Here's how the part is built. I have some questions about the finished solid (model axes, mm). Face numbers are marked on the shaded views. A direction names the side the tool comes from. Coordinates: 2 decimals unless noted, no trailing zeros. Order: outer loops, then holes, each group sorted by start corner. A loop starts at its lowest first (then second) coordinate and runs counter-clockwise, first axis right, second up. Notation, with made-up numbers: (81.25, -35) - (110.25, -35) arc R21 cw to (110.25, -29) - close; hole circle Ø4 at (17.5, 69). An arc over 180 degrees is marked (long way). Answer as CSV lines item,"result". Start each with the question number.
Q1. For pin 1 Ø1.2 at (y, z) = (0.5, 4) entering from -X; pin 2 Ø2.5 at (y, z) = (-3.5, 6) entering from +X (3 decimals); pin 3 Ø3.5 at (y, z) = (-3, 1.5) entering from -X (3 decimals), each with a flat end and sliding along its axis, tell me the tip position at first contact or that it passes through.
Q2. Suppose I cut it at D-D (x = 1.5). Please give me the cut outline in (y, z), then the cut area to 3 significant figures.
Q3. Suppose I cut it at A-A (x = 18.5). Please give me the cut outline in (y, z) (3 decimals), then the cut area to 3 significant figures.
Q4. Suppose I cut it at B-B (z = 4). Please give me the cut outline in (x, y).
Q5. I need wall thicknesses on line 1 (Y direction, x = 18.5, z = 1.25); line 2 (X direction, y = 8, z = 5); line 3 (Z direction, x = 13.25, y = 3.5) (3 decimals). Which ranges of each line are inside material? Lowest first, please.
Q6. Suppose I cut it at C-C (y = 1). Please give me the cut outline in (x, z), then the cut area to 3 significant figures.
Q7. For the marked faces 1, 2 and 3, which set-ups out of +Z, -Z, +X, -X, +Y, -Y let a thin tool reach every point of the face, with its end or its side?
Q8. Thinking about a two-plate mould opening in Y: for the marked faces 4, 5 and 6, which applies, released by +Y, released by -Y, zero draft, split by the parting line, or undercut?
Autodesk Inventor part; units mm, degrees
ref_plane "YZ Plane" through (0, 0, 0) normal (1, 0, 0) x (0, 1, 0)
ref_plane "XZ Plane" through (0, 0, 0) normal (0, 1, 0) x (-1, 0, 0)
ref_plane "XY Plane" through (0, 0, 0) normal (0, 0, 1) x (1, 0, 0)
sketch "Sketch1" plane through (0, 0, 0) normal (0, 0, 1) x (1, 0, 0)
  line L0 (0, 0) -> (25, 0)
  line L1 (25, 0) -> (25, 12)
  line L2 (25, 12) -> (0, 12)
  line L3 (0, 12) -> (0, 0)
  line L4 (10.625, 0) -> (14.375, 0)
  line L5 (14.375, 0) -> (14.375, -6)
  line L6 (14.375, -6) -> (10.625, -6) construction
  line L7 (10.625, -6) -> (10.625, 0)
  line L8 (0, -6) -> (25, -6)
  line L9 (25, -6) -> (25, -9)
  line L10 (25, -9) -> (0, -9)
  line L11 (0, -9) -> (0, -6)
  point P0 (14.375, 0)
  dimension "d0" = 25
  dimension "d1" = 12
  dimension "d2" = 6
  dimension "d3" = 3.75
  dimension "d4" = 10.625
  dimension "d28" = 0
  dimension "d29" = 3
extrude "Extrusion1" add sketch "Sketch1" along normal blind 8
sketch "Sketch2" plane through (0, 12, 0) normal (0, 1, 0) x (1, 0, 0)
  line L0 (0, 0) -> (10.625, 0)
  line L1 (0, 0) -> (25, 0)
  line L2 (25, 0) -> (25, -8)
  line L3 (25, -8) -> (0, -8)
  line L4 (0, -8) -> (0, 0)
  line L5 (2.75, -1.875) -> (22.25, -1.875)
  line L6 (22.25, -1.875) -> (22.25, -6.125)
  line L7 (22.25, -6.125) -> (2.75, -6.125)
  line L8 (2.75, -6.125) -> (2.75, -1.875)
  line L9 (5.05, -4.75) -> (10.8, -4.75)
  line L10 (10.8, -4.75) -> (10.8, -3.25)
  line L11 (10.8, -3.25) -> (5.05, -3.25)
  line L12 (5.05, -3.25) -> (5.05, -4.75)
  line L13 (14.2, -4.75) -> (19.95, -4.75)
  line L14 (19.95, -4.75) -> (19.95, -3.25)
  line L15 (19.95, -3.25) -> (14.2, -3.25)
  line L16 (14.2, -3.25) -> (14.2, -4.75)
  line L17 (2.95, -6) -> (22.05, -6) construction
  line L18 (22.05, -6) -> (22.05, -2) construction
  line L19 (22.05, -2) -> (2.95, -2) construction
  line L20 (2.95, -2) -> (2.95, -6) construction
  dimension "d7" = 25
  dimension "d8" = 8
  dimension "d9" = 19.5
  dimension "d10" = 4.25
  dimension "d11" = 1.875
  dimension "d12" = 2.75
  dimension "d13" = 1.5
  dimension "d14" = 19.1
  dimension "d15" = 4
  dimension "d16" = 2.95
  dimension "d17" = 2
  dimension "d18" = 2.1
  dimension "d20" = 2.1
  dimension "d21" = 1.25
  dimension "d22" = 5.75
  dimension "d23" = 5.75
extrude "Extrusion2" cut sketch "Sketch2" against normal blind 10 contours L5 L6 L7 L8 | L12 L11 L10 L9 | L16 L15 L14 L13
extrude "Extrusion3" cut sketch "Sketch2" against normal blind 18 contours L12 L11 L10 L9 | L16 L15 L14 L13
properties part number "fusebox"
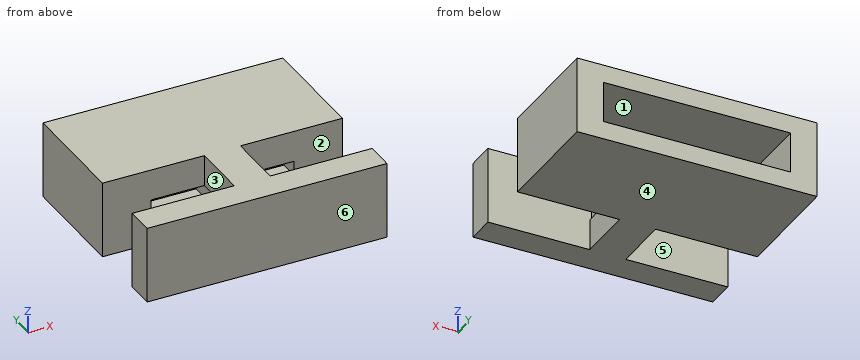
Here are the results:
1,pin 1,"stops at x = 0"
1,pin 2,"stops at x = 14.375"
1,pin 3,"stops at x = 10.625"
2,outline,"(-9, 0) - (-6, 0) - (-6, 8) - (-9, 8) - close; (0, 0) - (12, 0) - (12, 8) - (0, 8) - close"
2,area,"120 mm²"
3,outline,"(-9, 0) - (-6, 0) - (-6, 8) - (-9, 8) - close; (0, 0) - (12, 0) - (12, 1.875) - (2, 1.875) - (2, 3.25) - (0, 3.25) - close; (0, 4.75) - (2, 4.75) - (2, 6.125) - (12, 6.125) - (12, 8) - (0, 8) - close"
3,area,"74.5 mm²"
4,outline,"(0, -9) - (25, -9) - (25, -6) - (14.2, -6) - (14.2, 2) - (10.8, 2) - (10.8, -6) - (0, -6) - close; (0, 0) - (5.05, 0) - (5.05, 2) - (2.75, 2) - (2.75, 12) - (0, 12) - close; (19.95, 0) - (25, 0) - (25, 12) - (22.25, 12) - (22.25, 2) - (19.95, 2) - close"
5,line 1,"y = -9 to -6, 0 to 12"
5,line 2,"x = 0 to 2.75, 22.25 to 25"
5,line 3,"z = 0 to 1.875, 6.125 to 8"
6,outline,"(0, 0) - (25, 0) - (25, 8) - (0, 8) - close; hole (5.05, 3.25) - (10.8, 3.25) - (10.8, 4.75) - (5.05, 4.75) - close; hole (14.2, 3.25) - (19.95, 3.25) - (19.95, 4.75) - (14.2, 4.75) - close"
6,area,"183 mm²"
7,face 1,"+Y"
7,face 2,"+Z, -Z, +X"
7,face 3,"+Z, -Z, -X"
8,face 4,"zero draft"
8,face 5,"undercut"
8,face 6,"released by -Y"
